Part model, mm, in its own coordinate system. Face numbers are marked on the shaded views. A direction names the side the tool comes from. Coordinates: 2 decimals unless noted, no trailing zeros. Write each loop counter-clockwise with the first axis right and the second up, starting at its lowest first coordinate (ties: lowest second). Pieces come first, ordered by that corner, then holes. Notation, with made-up numbers: (-39.75, -36.75) - (14.25, -36.75) arc R17 cw to (14.25, -7.75) - close; hole circle Ø8 at (73, 82). An arc over 180 degrees is marked (long way). Use a Markdown table: item, result.
```python
from build123d import *

# Parameters (mm, degrees)
F0_R          = 38.1
F0_R_2        = 32.512
F1_DEPTH      = 38.1
F0_R_3        = 3.175
F2_DEPTH      = 11.176
F0_R_4        = 8.255
F3_DEPTH      = 11.176
F3_DEPTH_BACK = 12.7
F4_START      = -3.048
F4_DEPTH      = 9.652


with BuildPart() as f1:
    # F0 (on Top) → F1 (new body)
    with BuildSketch(Plane.XY):
        Circle(F0_R)
        Circle(F0_R_2, mode=Mode.SUBTRACT)
    extrude(amount=F1_DEPTH)

    # F0 (on Top) → F2 (join)
    with BuildSketch(Plane.XY):
        Circle(F0_R_2)
        with BuildLine():
            ThreePointArc((6.3494223473, 14.5499299262), (13.2818053133, 8.6953592576), (15.875, 0))
            ThreePointArc((15.875, 0), (-8.6950956004, -13.2819779212), (-6.35, 14.5496778315))
            Line((-6.35, 14.5496778315), (-6.35, 22.225))
            ThreePointArc((-6.35, 22.225), (0, 28.575), (6.35, 22.225))
            ThreePointArc((6.35, 22.225), (6.3498555852, 22.18217422), (6.3494223473, 22.139350388))
            Line((6.3494223473, 22.139350388), (6.3494223473, 14.5499299262))
        make_face(mode=Mode.SUBTRACT)
        with Locations((15.7154482119, 15.7154482119)):
            Circle(F0_R_3, mode=Mode.SUBTRACT)
        with BuildLine():
            ThreePointArc((-6.35, 22.225), (-4.4901280605, 17.7348719395), (0, 15.875))
            ThreePointArc((0, 15.875), (4.4597435444, 17.7046916568), (6.3494223473, 22.139350388))
            ThreePointArc((6.3494223473, 22.139350388), (6.3498555852, 22.18217422), (6.35, 22.225))
            ThreePointArc((6.35, 22.225), (0, 28.575), (-6.35, 22.225))
        make_face()
        with BuildLine():
            ThreePointArc((0, 15.875), (3.2431071076, 15.5402020994), (6.3494223473, 14.5499299262))
            Line((6.3494223473, 14.5499299262), (6.3494223473, 22.139350388))
            ThreePointArc((6.3494223473, 22.139350388), (4.4597435444, 17.7046916568), (0, 15.875))
        make_face()
        with BuildLine():
            Line((-6.35, 22.225), (-6.35, 14.5496778315))
            ThreePointArc((-6.35, 14.5496778315), (-3.2434155936, 15.5401377178), (0, 15.875))
            ThreePointArc((0, 15.875), (-4.4901280605, 17.7348719395), (-6.35, 22.225))
        make_face()
    extrude(amount=F2_DEPTH)

    # F0 (on Top) → F3 (join, two sides)
    with BuildSketch(Plane.XY) as f3_sk:
        with BuildLine():
            ThreePointArc((-6.35, 14.5496778315), (-8.6950956004, -13.2819779212), (15.875, 0))
            ThreePointArc((15.875, 0), (13.2818053133, 8.6953592576), (6.3494223473, 14.5499299262))
            ThreePointArc((6.3494223473, 14.5499299262), (3.2431071076, 15.5402020994), (0, 15.875))
            ThreePointArc((0, 15.875), (-3.2434155936, 15.5401377178), (-6.35, 14.5496778315))
        make_face()
        Circle(F0_R_4, mode=Mode.SUBTRACT)
    extrude(amount=F3_DEPTH)
    extrude(f3_sk.sketch, amount=-F3_DEPTH_BACK)

    # F0 (on Top) → F4 (join)
    with BuildSketch(Plane.XY.offset(F4_START)):
        with BuildLine():
            ThreePointArc((-6.35, 22.225), (-4.4901280605, 17.7348719395), (0, 15.875))
            ThreePointArc((0, 15.875), (4.4597435444, 17.7046916568), (6.3494223473, 22.139350388))
            ThreePointArc((6.3494223473, 22.139350388), (6.3498555852, 22.18217422), (6.35, 22.225))
            ThreePointArc((6.35, 22.225), (0, 28.575), (-6.35, 22.225))
        make_face()
        with BuildLine():
            Line((-6.35, 22.225), (-6.35, 14.5496778315))
            ThreePointArc((-6.35, 14.5496778315), (-3.2434155936, 15.5401377178), (0, 15.875))
            ThreePointArc((0, 15.875), (-4.4901280605, 17.7348719395), (-6.35, 22.225))
        make_face()
        with BuildLine():
            ThreePointArc((0, 15.875), (3.2431071076, 15.5402020994), (6.3494223473, 14.5499299262))
            Line((6.3494223473, 14.5499299262), (6.3494223473, 22.139350388))
            ThreePointArc((6.3494223473, 22.139350388), (4.4597435444, 17.7046916568), (0, 15.875))
        make_face()
    extrude(amount=-F4_DEPTH)


solid = f1.part
```
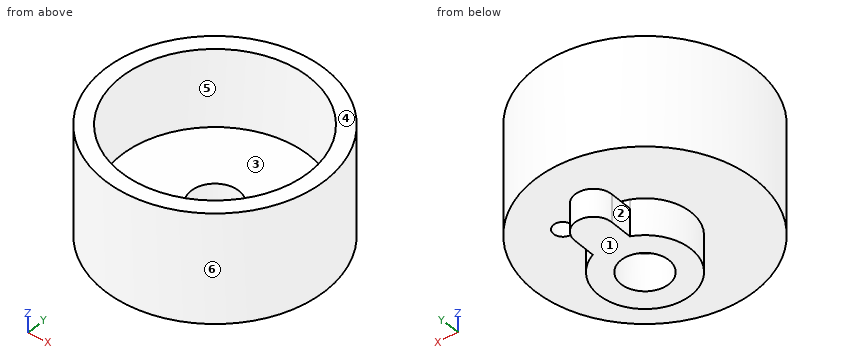
Item 1: Drill centre lines: probe 1 along Y at (x, z) = (0, -5.75) (3 decimals); probe 2 along Y at (x, z) = (0, 25.25); probe 3 along Z at (x, y) = (3.5, 34.5). Where is each one in solid material? Low to high.
From the geometry:
| item | result |
|---|---|
| probe 1 | -15.875 to -8.255, 8.255 to 28.575 |
| probe 2 | -38.1 to -32.51, 32.51 to 38.1 |
| probe 3 | 0 to 38.1 |
Item 2: Drop flat-ended pins along their axis: P1, Ø5, axis at x = 15.72, y = 15.72, coming from the -Z side; P2, Ø8, axis at y = -27.5, z = -1.5, coming from the -X side; P3, Ø14, axis at x = -1.5, y = 21, coming from the +Z side; P4, Ø2.5, axis at y = 19.5, z = -5.5, coming from the +X side. Give the stop position or say it passes through.
From the geometry:
| item | result |
|---|---|
| P1 | through |
| P2 | x = -29.76 |
| P3 | z = 11.18 |
| P4 | x = 6.35 |
Item 3: Band-saw the part on B-B, the plane x = -5. Give the cut face in (y, z).
From the geometry:
| item | result |
|---|---|
| outline | (-37.77, 0) - (-15.07, 0) - (-15.07, -12.7) - (-6.57, -12.7) - (-6.57, 11.18) - (-32.13, 11.18) - (-32.13, 38.1) - (-37.77, 38.1) - close; (6.57, -12.7) - (26.14, -12.7) - (26.14, -3.05) - (15.07, -3.05) - (15.07, 0) - (37.77, 0) - (37.77, 38.1) - (32.13, 38.1) - (32.13, 11.18) - (6.57, 11.18) - close |
Item 4: Band-saw the part on A-A, the plane z = -1. Give the cut face in (x, y) (3 decimals), then the cut area to 3 significant figures.
From the geometry:
| item | result |
|---|---|
| outline | circle Ø31.75 at (0, 0); hole circle Ø16.51 at (0, 0) |
| area | 578 mm^2 |
Item 5: Two-plate mould, pull along Y, no slides. Class the marked faces 4, 5 and 6: pulls with the +Y half, pulls with the -Y half, needs draft (parallel to the pull), parting line crosses it, or undercut.
From the geometry:
| item | result |
|---|---|
| face 4 | needs draft |
| face 5 | undercut |
| face 6 | parting line crosses it |
Item 6: Band-saw the part on D-D, the plane z = 10. Give the cut face in (x, y) (3 decimals), then the cut area to 3 significant figures.
From the geometry:
| item | result |
|---|---|
| outline | circle Ø76.2 at (0, 0); hole circle Ø16.51 at (0, 0); hole circle Ø6.35 at (15.715, 15.715) |
| area | 4,310 mm^2 |
Item 7: Which spindle directions (+Z, -Z, +X, -X, +Y, -Y) get a long thin tool onto all of the face, cutting with end or side? Do the marked faces 1, 2 and 3. Say none if no direction does.
From the geometry:
| item | result |
|---|---|
| face 1 | -Z, +X, -X, +Y, -Y |
| face 2 | -Z, -X, +Y |
| face 3 | +Z |
Item 8: Band-saw the part on C-C, the plane x = 20. Give the cut face in (y, z), then the cut area to 3 significant figures.
From the geometry:
| item | result |
|---|---|
| outline | (-32.43, 0) - (32.43, 0) - (32.43, 38.1) - (25.63, 38.1) - (25.63, 11.18) - (-25.63, 11.18) - (-25.63, 38.1) - (-32.43, 38.1) - close |
| area | 1,090 mm^2 |
